from build123d import *

# Parameters (mm, degrees)
F1_DEPTH = 35


with BuildPart() as f1:
    # F0 (on Right) → F1 (new body, symmetric)
    with BuildSketch(Plane.YZ):
        with BuildLine():
            Line((-17.5, -5), (-17.5, 0))
            Line((-17.5, 0), (0, 0))
            Line((0, 0), (17.5, 0))
            Line((17.5, 0), (17.5, -5))
            Line((17.5, -5), (45, -5))
            Line((45, -5), (45, 47.5))
            Line((45, 47.5), (25, 47.5))
            Line((25, 47.5), (25, 57.5))
            ThreePointArc((25, 57.5), (12.5224797864, 58.6246631061), (0, 59))
            ThreePointArc((0, 59), (-12.5224797864, 58.6246631061), (-25, 57.5))
            Line((-25, 57.5), (-25, 47.5))
            Line((-25, 47.5), (-45, 47.5))
            Line((-45, 47.5), (-45, -5))
            Line((-45, -5), (-17.5, -5))
        make_face()
    extrude(amount=F1_DEPTH, both=True)


solid = f1.part
Here's how the part is built. I have some questions about the finished solid (model axes, mm). A direction names the side the tool comes from. Coordinates: 2 decimals unless noted, no trailing zeros. Order: outer loops, then holes, each group sorted by start corner. A loop starts at its lowest first (then second) coordinate and runs counter-clockwise, first axis right, second up. Notation, with made-up numbers: (-20.75, -4.5) -> (-3.75, -4.5) arc R7 cw to (-3.75, 5.5) -> close; hole circle Ø9 at (26, 2). An arc over 180 degrees is marked (long way). Answer in a Markdown table with one row per item.
(1) On a 3-axis mill with a long thin cutter (end or side, diameter ignored), from which of +Z, -Z, +X, -X, +Y, -Y can I reach the whole of each face in a straight line? I mean faces 5 (the face through (0, 0, 59)), 6 (the face through (0, -17.5, -3)), 7 (the face through (0, -25, 53)), 8 (the face through (0, 35, 47.5)). Say none if no direction works.
Answer key:
| item | result |
|---|---|
| face 5 | +Z, +X, -X |
| face 6 | -Z, +X, -X |
| face 7 | +Z, +X, -X, -Y |
| face 8 | +Z, +X, -X, +Y |
(2) Will these pins go through, and if not, where does the flat tip stop? pin 1 Ø6 at (x, y) = (-24, 33) entering from +Z; pin 2 Ø1 at (x, y) = (17.5, -24.5) entering from +Z; pin 3 Ø11 at (x, z) = (-9, 53.5) entering from -Y.
Answer key:
| item | result |
|---|---|
| pin 1 | z = 47.5 |
| pin 2 | z = 57.62 |
| pin 3 | y = -25 |
(3) Please list where these lines run through material, in increasing order: probe 1 along Z at (x, y) = (31.5, -41); probe 2 along Y at (x, z) = (-28, 49); probe 3 along Z at (x, y) = (-30.5, 15).
Answer key:
| item | result |
|---|---|
| probe 1 | -5 to 47.5 |
| probe 2 | -25 to 25 |
| probe 3 | 0 to 58.46 |
(4) I want a section at A-A on x = -26.5. List the corners of the cut face in (y, z) for me, then the cut area to 3 significant figures.
Answer key:
| item | result |
|---|---|
| outline | (-45, -5) -> (-17.5, -5) -> (-17.5, 0) -> (17.5, 0) -> (17.5, -5) -> (45, -5) -> (45, 47.5) -> (25, 47.5) -> (25, 57.5) arc R209.08 ccw to (-25, 57.5) -> (-25, 47.5) -> (-45, 47.5) -> close |
| area | 5,100 mm^2 |
(5) I want a section at B-B on y = -22. List the corners of the cut face in (x, z) for me.
Answer key:
| item | result |
|---|---|
| outline | (-35, -5) -> (35, -5) -> (35, 57.84) -> (-35, 57.84) -> close |
(6) Thinking about a two-plate mould opening in Y: for faces 1 (the face through (0, 0, 0)), 2 (the face through (-35, -1, 27)), 3 (the face through (0, 25, 52)), 4 (the face through (0, 17.5, -2)), which applies, +Y half, -Y half, draft (parallel to the pull), parting line (faces both ways), or undercut?
Answer key:
| item | result |
|---|---|
| face 1 | undercut |
| face 2 | draft |
| face 3 | +Y half |
| face 4 | undercut |
(7) I want a section at C-C on y = -4.5. List the corners of the cut face in (x, z) for me, then the cut area to 3 significant figures.
Answer key:
| item | result |
|---|---|
| outline | (-35, 0) -> (35, 0) -> (35, 58.95) -> (-35, 58.95) -> close |
| area | 4,130 mm^2 |
